The listing builds one solid part. Answer for the finished solid, in the listing's coordinates (mm). Give positions to 0.01 mm unless a question says otherwise; leave off trailing zeros. Loops run counter-clockwise (first coordinate to the right, second up) from the corner with the lowest first, then second, coordinate; pieces in that order, holes last. Notation, with made-up numbers: (19.5, 35.25) - (48.5, 35.25) arc R23 cw to (48.5, 70.25) - close; hole circle Ø4 at (65.25, -35.75). An arc over 180 degrees is marked (long way). Answer as CSV lines item,"result". Start each with the question number.
1) A cutting plane is placed at A-A (y = 0). Determine the outline of the cut face in (x, z).
2) Find the intervals of material crossed by line 1 along Y through (x, z) = (0, 4); line 2 along Y through (x, z) = (1, 0.5), in increasing order.
3) A cutting plane is placed at C-C (z = 1.25). Determine the outline of the cut face in (x, y), and give its area (3 significant figures).
4) For a pull along Y with two mould halves and no side action, classify faces 1 (the face through (-3, 3, 0)), 2 (the face through (-0.867, -3.905, 3.131)), 3 (the face through (0, -6.35, 3)) as pulls with the +Y half, pulls with the -Y half, needs draft (parallel to the pull), parting line crosses it, or undercut.
```python
from build123d import *

# Parameters (mm, degrees)
CYLINDER035_R     = 4
CYLINDER035_DEPTH = 10
BOX014_W          = 12.7
BOX014_H          = 12.7
BOX014_DEPTH      = 6.35


with BuildPart() as cylinder035:
    # Cylinder035 → Cylinder035 (new body)
    with BuildSketch(Plane(origin=(6.35, 6.35, 0), x_dir=(1, 0, 0), z_dir=(0, 0, 1))):
        Circle(CYLINDER035_R)
    extrude(amount=CYLINDER035_DEPTH)


with BuildPart() as m8_nut001:
    # Box014 → Box014 (new body)
    with BuildSketch(Plane.XY):
        with Locations((6.35, 6.35)):
            Rectangle(BOX014_W, BOX014_H)
    extrude(amount=BOX014_DEPTH)

    # Cut012: cut Cylinder035
    add(cylinder035.part, mode=Mode.SUBTRACT)


with BuildPart() as m8_nut001_1:
    # Cut012 placement: moved
    add(m8_nut001.part.moved(Location((-6.35, -6.35, 0))))


solid = m8_nut001_1.part
```
Ans:
1,outline,"(-6.35, 0) - (-4, 0) - (-4, 6.35) - (-6.35, 6.35) - close; (4, 0) - (6.35, 0) - (6.35, 6.35) - (4, 6.35) - close"
2,line 1,"-6.35 to -4, 4 to 6.35"
2,line 2,"-6.35 to -3.87, 3.87 to 6.35"
3,outline,"(-6.35, -6.35) - (6.35, -6.35) - (6.35, 6.35) - (-6.35, 6.35) - close; hole circle Ø8 at (0, 0)"
3,area,"111 mm2"
4,face 1,"needs draft"
4,face 2,"undercut"
4,face 3,"pulls with the -Y half"
